Read the model definition and answer for the solid it produces. Units are mm, in the model's axes. Face numbers are marked on the shaded views. A direction names the side the tool comes from. Coordinates: 2 decimals unless noted, no trailing zeros. Order: outer loops, then holes, each group sorted by start corner. A loop starts at its lowest first (then second) coordinate and runs counter-clockwise, first axis right, second up. Notation, with made-up numbers: (-38, 38.25) - (-17, 38.25) arc R8 cw to (-17, 49.25) - close; hole circle Ø6 at (13.5, 38.5). An arc over 180 degrees is marked (long way). Answer as a JSON object with one key per item and string values. Group by question number.
from build123d import *

# Parameters (mm, degrees)
PAD002_DEPTH    = 2.9
PAD003_DEPTH    = 4.9
POCKET005_DEPTH = 4.1
POCKET006_DEPTH = 11
SKETCH011_W     = 10
SKETCH011_H     = 3.6
POCKET007_DEPTH = 5
PAD004_DEPTH    = 2


with BuildPart() as part:
    # Sketch008 (on Face1 of ReferencePocket001) → Pad002 (new body)
    with BuildSketch(Plane.XY.offset(3.9)):
        with BuildLine():
            Line((0.2, 0.2), (18.2000000001, 0.2))
            Line((18.2000000001, 0.2), (18.2000000001, 25.6999686791))
            ThreePointArc((18.2000000001, 25.6999686791), (9.2000000001, 34.6999686791), (0.2, 25.6999686791))
            Line((0.2, 0.2), (0.2, 25.6999686791))
        make_face()
        with BuildLine():
            Line((0.8, 0.8), (17.6000000001, 0.8))
            Line((17.6000000001, 0.8), (17.6000000001, 25.6999686791))
            ThreePointArc((17.6000000001, 25.6999686791), (9.2000000001, 34.0999686791), (0.8, 25.6999686791))
            Line((0.8, 0.8), (0.8, 25.6999686791))
        make_face(mode=Mode.SUBTRACT)
    extrude(amount=-PAD002_DEPTH)

    # Sketch009 (on Face9 of Pad002) → Pad003 (join)
    with BuildSketch(Plane.XY.offset(3.9)):
        with BuildLine():
            Line((-0.86, -0.86), (19.26, -0.86))
            Line((19.26, -0.86), (19.26, 25.7000002895))
            ThreePointArc((19.26, 25.7000002895), (9.1999999842, 35.7600002578), (-0.86, 25.7000002578))
            Line((-0.86, -0.86), (-0.86, 25.7000002578))
        make_face()
    extrude(amount=PAD003_DEPTH)

    # Pad003 Face16 → Pocket005 (cut)
    with BuildSketch(Plane(origin=(9.2000000001, 16.6044557437, 3.9), x_dir=(0, -1, 0), z_dir=(0, 0, -1))):
        with BuildLine():
            Line((15.8044557437, 8.4000000001), (-9.0955129353, 8.4000000001))
            ThreePointArc((-9.0955129353, 8.4000000001), (-17.4955129354, 0), (-9.0955129353, -8.4000000001))
            Line((-9.0955129353, -8.4000000001), (15.8044557437, -8.4000000001))
            Line((15.8044557437, -8.4000000001), (15.8044557437, 8.4000000001))
        make_face()
    extrude(amount=-POCKET005_DEPTH, mode=Mode.SUBTRACT)

    # Sketch010 (on Face8 of Pocket005) → Pocket006 (cut)
    with BuildSketch(Plane.YZ.offset(18.2000000001)):
        Polygon((0.81, 1), (5.2, 1), (20.2, 1), (20.2, 2.5), (5.2, 2.5), (5.2, 5.5), (0.81, 5.5), (0.81, 1.8), (0.2, 1.8), (0.2, 1), align=None)
    extrude(amount=-POCKET006_DEPTH, mode=Mode.SUBTRACT)

    # Sketch011 (on Face12 of Pocket006) → Pocket007 (cut)
    with BuildSketch(Plane(origin=(0.2, 0, 0), x_dir=(0, -1, 0), z_dir=(-1, 0, 0))):
        with Locations((-14, 1.8)):
            Rectangle(SKETCH011_W, SKETCH011_H)
    extrude(amount=-POCKET007_DEPTH, mode=Mode.SUBTRACT)

    # Sketch012 (on Face12 of Pocket007) → Pad004 (join)
    with BuildSketch(Plane(origin=(10.2, 0, 0), x_dir=(0, -1, 0), z_dir=(-1, 0, 0))):
        Polygon((-0.2, 2.5), (0, 2.7), (0, 3.1), (-0.2, 3.3), align=None)
        Polygon((-34.8999686791, 2.6), (-34.8999686791, 3), (-34.4999686791, 3.4), (-34.4999686791, 2.2), align=None)
    extrude(amount=PAD004_DEPTH)


solid = part.part
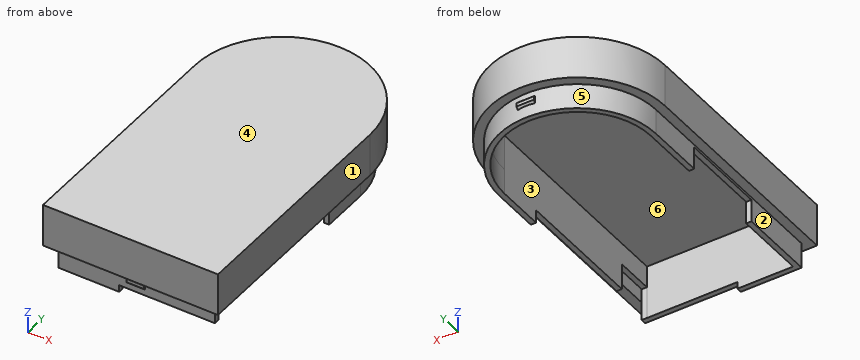
1. For a pull along Y with two mould halves and no side action, classify the marked faces 4, 5 and 6 as pulls with the +Y half, pulls with the -Y half, needs draft (parallel to the pull), parting line crosses it, or undercut.
2. A cutting plane is placed at C-C on x = 16.5. Write down the section's boundary in (y, z).
3. For the marked faces 1, 2 and 3, determine the directions among +Z, -Z, +X, -X, +Y, -Y from which every point of the face is accessible in a straight line to the end or side of a thin tool.
4. Straight lines are drawn through the part: L1, parallel to X at y = 8, z = 4.5; L2, parallel to X at y = 9.5, z = 3.75; L3, parallel to Y at x = 9.5, z = 4.5. For each, find the intervals that lie inside material, in ascending order.
5. A cutting plane is placed at B-B on y = 19.5. Write down the section's boundary in (x, z).
6. Given pin 1 (4 mm diameter, centred on x = 7, z = 2.5, fed in from +Y); pin 2 (6 mm diameter, centred on x = 13.5, y = 10.5, fed in from -Z); pin 3 (0.7 mm diameter, centred on x = 18, z = 2, fed in from -Y), each flat-ended and moving along its own axis, determine where each tip first touches the part or whether it passes through.
7. A cutting plane is placed at A-A on z = 7. Write down the section's boundary in (x, y), and give its area (3 significant figures).
Derived:
{
 "1": {"face 4": "needs draft", "face 5": "pulls with the +Y half", "face 6": "undercut"},
 "2": {"outline": "(-0.86, 3.9) - (0.2, 3.9) - (0.2, 1.8) - (0.8, 1.8) - (0.8, 8) - (29.86, 8) - (29.86, 1) - (30.96, 1) - (30.96, 3.9) - (32.62, 3.9) - (32.62, 8.8) - (-0.86, 8.8) - close"},
 "3": {"face 1": "+Z, -Z, +X, +Y, -Y", "face 2": "-Z, -X, +Y, -Y", "face 3": "-Z"},
 "4": {"L1": "x = -0.86 to 0.8, 17.6 to 19.26", "L2": "x = 0.2 to 0.8, 17.6 to 18.2", "L3": "y = -0.86 to 0.8, 34.09 to 35.76"},
 "5": {"outline": "(-0.86, 3.9) - (0.2, 3.9) - (0.2, 1) - (0.8, 1) - (0.8, 8) - (17.6, 8) - (17.6, 2.5) - (18.2, 2.5) - (18.2, 3.9) - (19.26, 3.9) - (19.26, 8.8) - (-0.86, 8.8) - close"},
 "6": {"pin 1": "stops at y = 35.73", "pin 2": "stops at z = 8", "pin 3": "stops at y = 0.2"},
 "7": {"outline": "(-0.86, -0.86) - (19.26, -0.86) - (19.26, 25.7) arc R10.06 ccw to (-0.86, 25.7) - close; hole (0.8, 0.8) - (17.6, 0.8) - (17.6, 25.7) arc R8.4 ccw to (0.8, 25.7) - close", "area": "164 mm2"}
}
